from build123d import *

# Parameters (mm, degrees)
BOSS_EXTRUDE1_DEPTH = 1.27


with BuildPart() as part:
    # Sketch1 → Boss-Extrude1 (new body, symmetric)
    with BuildSketch(Plane(origin=(0, 0, 0), x_dir=(1, 0, 0), z_dir=(0, 1, 0))):
        Polygon((67.5, -32.5), (67.5, 32.5), (-2.5, 32.5), (-2.5, 62.5), (-67.5, 62.5), (-67.5, -62.5), (-2.5, -62.5), (-2.5, -32.5), align=None)
    extrude(amount=BOSS_EXTRUDE1_DEPTH, both=True)


solid = part.part
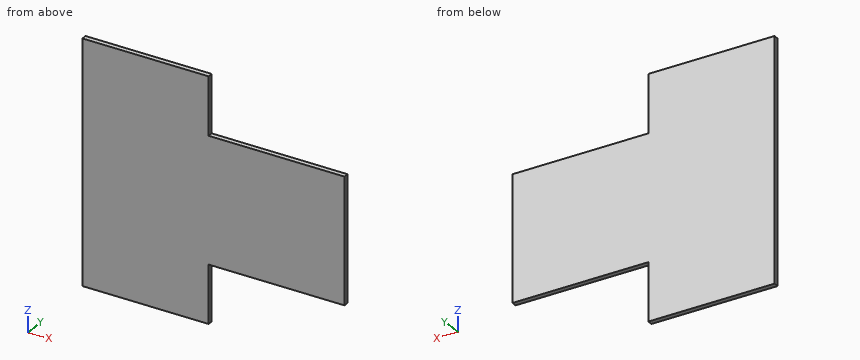
Input: part model. Units: mm. Frame: model coordinates. Round coordinates to 2 decimals unless told otherwise and drop trailing zeros. Write each loop counter-clockwise with the first axis right and the second up, starting at its lowest first coordinate (ties: lowest second). Pieces come first, ordered by that corner, then holes.
1) Cut plane B-B (x = 39.5). Return the cut outline in (y, z), then the cut area to 3 significant figures.
2) Cut plane C-C (z = -41.5). Return the cut outline in (x, y).
3) Cut plane A-A (y = -0.65). Return the cut outline in (x, z).
4) Contact query for a flat-ended pin moving along its axis: P1, Ø1.3, axis at y = 0, z = -51, coming from the +X side. Output: stop coordinate, or through.
5) Ray query, L1, parallel to X at y = -0.05, z = -46.5; L2, parallel to Z at x = 41, y = -0.9. Return the intervals inside material, ascending.
Geometry says:
1. outline: (-1.27, -32.5) - (1.27, -32.5) - (1.27, 32.5) - (-1.27, 32.5) - close
1. area: 165 mm2
2. outline: (-67.5, -1.27) - (-2.5, -1.27) - (-2.5, 1.27) - (-67.5, 1.27) - close
3. outline: (-67.5, -62.5) - (-2.5, -62.5) - (-2.5, -32.5) - (67.5, -32.5) - (67.5, 32.5) - (-2.5, 32.5) - (-2.5, 62.5) - (-67.5, 62.5) - close
4. P1: stops at x = -2.5
5. L1: x = -67.5 to -2.5
5. L2: z = -32.5 to 32.5
